For this review, take the finished solid that the model builds, in its own axes (mm). A direction names the side the tool comes from. Round coordinates to 2 decimals unless told otherwise and drop trailing zeros. Loops run counter-clockwise (first coordinate to the right, second up) from the corner with the lowest first, then second, coordinate; pieces in that order, holes last.
1) Take a section at B-B (z = -15.5). State the section outline as (x, y) points, then the cut area to 3 significant figures.
2) Take a section at A-A (x = 41). State the section outline as (y, z) points.
3) Take a section at D-D (y = 7.25). Give the number of separate pieces and of enclosed holes in the cut face, then the cut area to 3 significant figures.
4) Take a section at C-C (x = 14). State the section outline as (y, z) points, then the cut area to 3 significant figures.
5) Wall thickness on L1, parallel to X at y = 2.5, z = 11.25; L2, parallel to Z at x = 5.5, y = 4.5; L3, parallel to X at y = 8, z = -10: over which ranges is each line inside the solid? List them lowest first.
6) Insertion check: pin 1 (6 mm diameter, centred on x = -4, y = 5.5, fed in from +Z); pin 2 (1 mm diameter, centred on y = 9, z = -19.5, fed in from +X); pin 3 (3 mm diameter, centred on x = 26, y = 5, fed in from +Z). Each pin has a flat end and moves straight along its axis. Give the tip position at first contact, or say it passes through.
7) Mouldability with a two-part tool opening along Z and no side actions: class faces 1 (the cylindrical face through (-4.071, 5.83, 27.166)), 2 (the flat face through (-45, 5, 25.25)), 3 (the cylindrical face through (24, 5.67, 12.68)) as pulls with the +Z half, pulls with the -Z half, needs draft (parallel to the pull), parting line crosses it, or undercut.
8) Tool access review of faces 4 (the cylindrical face through (19.14, 5.83, 10.26)), 5 (the flat face through (54.25, 5, 20)), 6 (the flat face through (-30, 6, 26.75)): name each direction out of +Z, -Z, +X, -X, +Y, -Y from which nothing blocks a thin tool from reaching the whole face with its end or side.
```python
from build123d import *

# Parameters (mm, degrees)
BOSS_EXTRUDE1_DEPTH = 11.5
SKETCH2_W           = 32.4
SKETCH2_H           = 32.4
CUT_EXTRUDE1_DEPTH  = 8.7
SKETCH3_R           = 2
SKETCH3_W           = 108.5
SKETCH3_H           = 10.5
CUT_EXTRUDE2_DEPTH  = 10.7
CUT_EXTRUDE3_REACH  = 66.561
SKETCH5_W           = 32.8
SKETCH5_H           = 40
CUT_EXTRUDE4_DEPTH  = 10.7
SKETCH6_W           = 32.8
SKETCH6_H           = 1.5
BOSS_EXTRUDE2_DEPTH = 7.7
SKETCH8_R           = 2
SKETCH8_R_2         = 1.25
BOSS_EXTRUDE5_DEPTH = 11.5
FILLET1_R           = 2
SKETCH9_R           = 0.5
BOSS_EXTRUDE6_DEPTH = 10.7


with BuildPart() as part:
    # Sketch1 → Boss-Extrude1 (new body)
    with BuildSketch(Plane(origin=(0, 0, 0), x_dir=(1, 0, 0), z_dir=(0, 1, 0))):
        with BuildLine():
            Line((3.464101615, -26.75), (55.75, -26.75))
            Line((55.75, -26.75), (55.75, -13.25))
            Line((55.75, -13.25), (17.9, -13.25))
            Line((17.9, -13.25), (17.9, 26.75))
            Line((17.9, 26.75), (-17.9, 26.75))
            Line((-17.9, 26.75), (-17.9, -13.25))
            Line((-17.9, -13.25), (-55.75, -13.25))
            Line((-55.75, -13.25), (-55.75, -26.75))
            Line((-55.75, -26.75), (-3.464101615, -26.75))
            ThreePointArc((-3.464101615, -26.75), (0, -30.75), (3.464101615, -26.75))
        make_face()
    extrude(amount=BOSS_EXTRUDE1_DEPTH)

    # Sketch2 → Cut-Extrude1 (cut)
    with BuildSketch(Plane(origin=(0, 11.5, 0), x_dir=(1, 0, 0), z_dir=(0, 1, 0))):
        with Locations((0, 8.85)):
            Rectangle(SKETCH2_W, SKETCH2_H)
    extrude(amount=-CUT_EXTRUDE1_DEPTH, mode=Mode.SUBTRACT)

    # Sketch3 → Cut-Extrude2 (cut)
    with BuildSketch(Plane.XZ):
        with Locations((0, 27.25)):
            Circle(SKETCH3_R)
        with BuildLine():
            Line((-2, 27.25), (-2, 25.25))
            Line((-2, 25.25), (-1e-08, 25.25))
            ThreePointArc((-1e-08, 25.25), (-1.414213566, 25.835786441), (-2, 27.25))
        make_face()
        with BuildLine():
            ThreePointArc((2, 27.25), (1.414213559, 25.835786434), (-1e-08, 25.25))
            Line((-1e-08, 25.25), (2, 25.25))
            Line((2, 25.25), (2, 27.25))
        make_face()
        with Locations((0, 20)):
            Rectangle(SKETCH3_W, SKETCH3_H)
    extrude(amount=-CUT_EXTRUDE2_DEPTH, mode=Mode.SUBTRACT)

    # Sketch4 → Cut-Extrude3 (cut, up to next)
    with BuildSketch(Plane.XZ.offset(-10.7), mode=Mode.PRIVATE) as cut_extrude3_sk1:
        with BuildLine():
            Line((51, 16.75), (-51, 16.75))
            ThreePointArc((-51, 16.75), (-52.75, 18.5), (-51, 20.25))
            Line((-51, 20.25), (51, 20.25))
            ThreePointArc((51, 20.25), (52.75, 18.5), (51, 16.75))
        make_face()
    cut_extrude3_tool1 = extrude(cut_extrude3_sk1.sketch, amount=-CUT_EXTRUDE3_REACH, mode=Mode.PRIVATE) & part.part
    add(cut_extrude3_tool1.solids().sort_by_distance((0, 10.7, 18.5))[0], mode=Mode.SUBTRACT)

    # Sketch5 → Cut-Extrude4 (cut)
    with BuildSketch(Plane.XZ):
        with Locations((0, -5.25)):
            Rectangle(SKETCH5_W, SKETCH5_H)
    extrude(amount=-CUT_EXTRUDE4_DEPTH, mode=Mode.SUBTRACT)

    # Sketch6 → Boss-Extrude2 (add)
    with BuildSketch(Plane.XZ.offset(-10.7)):
        with Locations((0, 8.1)):
            Rectangle(SKETCH6_W, SKETCH6_H)
    extrude(amount=BOSS_EXTRUDE2_DEPTH)

    # Sketch8 → Boss-Extrude5 (add)
    # profile 1 of 10: a face of its own
    with BuildSketch(Plane(origin=(0, 11.5, 0), x_dir=(1, 0, 0), z_dir=(0, 1, 0))):
        with BuildLine():
            Line((-17.9, -7.75), (-19.9, -7.75))
            ThreePointArc((-19.9, -7.75), (-18.851902827, -7.910614979), (-17.9, -8.377718677))
            Line((-17.9, -8.377718677), (-17.9, -7.75))
        make_face()
    # profile 2 of 10: a face of its own
    with BuildSketch(Plane(origin=(0, 11.5, 0), x_dir=(1, 0, 0), z_dir=(0, 1, 0))):
        with BuildLine():
            ThreePointArc((-17.9, -8.377718677), (-18.851902827, -7.910614979), (-19.9, -7.75))
            ThreePointArc((-19.9, -7.75), (-22.374873734, -8.775126266), (-23.4, -11.25))
            ThreePointArc((-23.4, -11.25), (-23.239385021, -12.298097173), (-22.772281323, -13.25))
            Line((-22.772281323, -13.25), (-19.9, -13.25))
            ThreePointArc((-19.9, -13.25), (-21.314213562, -9.835786438), (-17.9, -11.25))
            Line((-17.9, -11.25), (-17.9, -8.377718677))
        make_face()
    # profile 3 of 10: a face of its own
    with BuildSketch(Plane(origin=(0, 11.5, 0), x_dir=(1, 0, 0), z_dir=(0, 1, 0))):
        with Locations((-19.9, -11.25)):
            Circle(SKETCH8_R)
        with Locations(Location((-19.9, -11.25, 0), (0, 0, 270))):
            Circle(SKETCH8_R_2, mode=Mode.SUBTRACT)
    # profile 4 of 10: a face of its own
    with BuildSketch(Plane(origin=(0, 11.5, 0), x_dir=(1, 0, 0), z_dir=(0, 1, 0))):
        with BuildLine():
            Line((-17.9, -13.25), (-17.9, -11.25))
            ThreePointArc((-17.9, -11.25), (-18.485786438, -12.664213562), (-19.9, -13.25))
            Line((-19.9, -13.25), (-17.9, -13.25))
        make_face()
    # profile 5 of 10: a face of its own
    with BuildSketch(Plane(origin=(0, 11.5, 0), x_dir=(1, 0, 0), z_dir=(0, 1, 0))):
        with BuildLine():
            ThreePointArc((-22.772281323, -13.25), (-23.239385021, -12.298097173), (-23.4, -11.25))
            Line((-23.4, -11.25), (-23.4, -13.25))
            Line((-23.4, -13.25), (-22.772281323, -13.25))
        make_face()
    # profile 6 of 10: a face of its own
    with BuildSketch(Plane(origin=(0, 11.5, 0), x_dir=(1, 0, 0), z_dir=(0, 1, 0))):
        with BuildLine():
            Line((17.9, -13.25), (19.9, -13.25))
            ThreePointArc((19.9, -13.25), (18.485786438, -12.664213562), (17.9, -11.25))
            Line((17.9, -11.25), (17.9, -13.25))
        make_face()
    # profile 7 of 10: a face of its own
    with BuildSketch(Plane(origin=(0, 11.5, 0), x_dir=(1, 0, 0), z_dir=(0, 1, 0))):
        with Locations((19.9, -11.25)):
            Circle(SKETCH8_R)
        with Locations(Location((19.9, -11.25, 0), (0, 0, 270))):
            Circle(SKETCH8_R_2, mode=Mode.SUBTRACT)
    # profile 8 of 10: a face of its own
    with BuildSketch(Plane(origin=(0, 11.5, 0), x_dir=(1, 0, 0), z_dir=(0, 1, 0))):
        with BuildLine():
            ThreePointArc((22.772281323, -13.25), (23.239385021, -12.298097173), (23.4, -11.25))
            ThreePointArc((23.4, -11.25), (22.374873734, -8.775126266), (19.9, -7.75))
            ThreePointArc((19.9, -7.75), (18.851902827, -7.910614979), (17.9, -8.377718677))
            Line((17.9, -8.377718677), (17.9, -11.25))
            ThreePointArc((17.9, -11.25), (19.9, -9.25), (21.9, -11.25))
            ThreePointArc((21.9, -11.25), (21.314213562, -12.664213562), (19.9, -13.25))
            Line((19.9, -13.25), (22.772281323, -13.25))
        make_face()
    # profile 9 of 10: a face of its own
    with BuildSketch(Plane(origin=(0, 11.5, 0), x_dir=(1, 0, 0), z_dir=(0, 1, 0))):
        with BuildLine():
            ThreePointArc((17.9, -8.377718677), (18.851902827, -7.910614979), (19.9, -7.75))
            Line((19.9, -7.75), (17.9, -7.75))
            Line((17.9, -7.75), (17.9, -8.377718677))
        make_face()
    # profile 10 of 10: a face of its own
    with BuildSketch(Plane(origin=(0, 11.5, 0), x_dir=(1, 0, 0), z_dir=(0, 1, 0))):
        with BuildLine():
            Line((23.4, -13.25), (23.4, -11.25))
            ThreePointArc((23.4, -11.25), (23.239385021, -12.298097173), (22.772281323, -13.25))
            Line((22.772281323, -13.25), (23.4, -13.25))
        make_face()
    extrude(amount=-BOSS_EXTRUDE5_DEPTH)

    # Fillet1
    fillet1_edges = [part.edges().sort_by_distance(p)[0] for p in [
        (55.75, 5.75, 26.75),
        (55.75, 5.75, 13.25),
        (-55.75, 5.75, 26.75),
        (-55.75, 5.75, 13.25),
        (-17.9, 5.75, -26.75),
        (17.9, 5.75, -26.75),
        (-17.9, 5.75, 7.75),
        (-23.4, 5.75, 13.25),
        (23.4, 5.75, 13.25),
        (17.9, 5.75, 7.75),
        (3.464101615, 5.75, 26.75),
        (-3.464101615, 5.75, 26.75),
    ]]
    fillet(fillet1_edges, radius=FILLET1_R - 0.0001)  # a hair under: the kernel refuses the full size

    # Sketch9 → Boss-Extrude6 (add)
    with BuildSketch(Plane.XZ.offset(-10.7)):
        with Locations((-35.325, 25.25)):
            Circle(SKETCH9_R)
        with Locations((-44.7875, 14.75)):
            Circle(SKETCH9_R)
        with Locations((35.325, 25.25)):
            Circle(SKETCH9_R)
        with Locations((44.7875, 14.75)):
            Circle(SKETCH9_R)
    extrude(amount=BOSS_EXTRUDE6_DEPTH)


solid = part.part
```
Response:
1. outline: (-17.9, 0) - (-16.4, 0) - (-16.4, 10.7) - (-16.2, 10.7) - (-16.2, 11.5) - (-17.9, 11.5) - close; (16.2, 10.7) - (16.4, 10.7) - (16.4, 0) - (17.9, 0) - (17.9, 11.5) - (16.2, 11.5) - close
1. area: 34.8 mm2
2. outline: (0, 13.25) - (11.5, 13.25) - (11.5, 16.75) - (10.7, 16.75) - (10.7, 14.75) - (0, 14.75) - close; (0, 25.25) - (10.7, 25.25) - (10.7, 20.25) - (11.5, 20.25) - (11.5, 26.75) - (0, 26.75) - close
3. separate pieces: 1
3. enclosed holes: 4
3. area: 590 mm2
4. outline: (0, -26.75) - (11.5, -26.75) - (11.5, -25.05) - (10.7, -25.05) - (10.7, -25.25) - (0, -25.25) - close; (0, 25.25) - (10.7, 25.25) - (10.7, 20.25) - (11.5, 20.25) - (11.5, 26.75) - (0, 26.75) - close; (3, 7.35) - (11.5, 7.35) - (11.5, 16.75) - (10.7, 16.75) - (10.7, 8.85) - (3, 8.85) - close
4. area: 57.7 mm2
5. L1: x = -23.4 to -21.15, -18.65 to -16.4, 16.4 to 18.65, 21.15 to 23.4
5. L2: z = -26.75 to -25.25, 7.35 to 8.85, 25.25 to 26.75
5. L3: x = -17.9 to -16.4, 16.4 to 17.9
6. pin 1: stops at z = 30.6
6. pin 2: stops at x = 17.9
6. pin 3: stops at z = 26.75
7. face 1: pulls with the +Z half
7. face 2: undercut
7. face 3: pulls with the -Z half
8. face 4: +Y, -Y
8. face 5: -Y
8. face 6: +Z, -X, +Y, -Y
